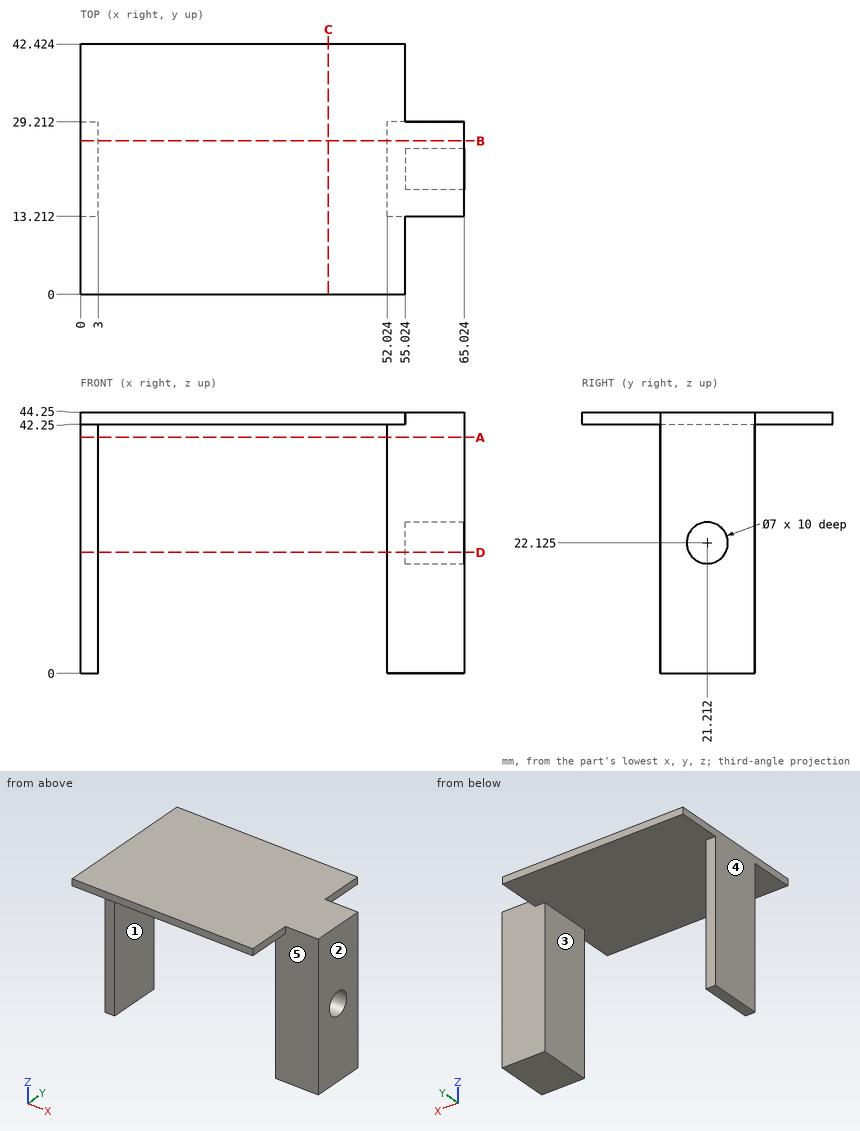
Check sheet for the drawn part. Datum: minimum x, y, z corner. Units: mm. A direction names the side the tool comes from. Give positions to 0.01 mm unless a question says otherwise; leave off trailing zeros. Write each loop counter-clockwise with the first axis right and the second up, starting at its lowest first coordinate (ties: lowest second). Pieces come first, ordered by that corner, then holes. Notation, with made-up numbers: (41.25, -9) -> (48.25, -9) arc R17 ccw to (48.25, 4) -> close; hole circle Ø9 at (63.5, -28). An arc over 180 degrees is marked (long way). Use one line per item in the form item = value. Start each with the question number.
1. Access from +Z, -Z, +X, -X, +Y, -Y to the whole of each face (thin tool, end or side, straight path). Record for the marked faces 1 and 2.
2. Section check A-A (z = 40). Record the cut outline in (x, y).
3. Thickness scan on line 1 along X through (y, z) = (22, 11.5); line 2 along Y through (x, z) = (60, 26); line 3 along Z through (x, y) = (44, 25). Record the ranges inside material, lowest first. Write a range as from..to.
4. Section check B-B (y = 26). Record the cut outline in (x, z).
5. Section check C-C (x = 42). Record the cut outline in (y, z).
6. Mould release check, pull along X, two halves, no side actions. Record for the marked faces 3, 4 and 5: pulls with the +X half, pulls with the -X half, needs draft (parallel to the pull), parting line crosses it, or undercut.
7. Section check D-D (z = 20.5). Record the cut outline in (x, y).
8. Go/stop test with flat-tipped pins: P1, Ø1.6, axis at y = 4, z = 43.5, coming from the +X side; P2, Ø6.5, axis at x = 57.5, z = 31.5, coming from the -Y side; P3, Ø1.5, axis at x = 2, z = 11.5, coming from the +Y side; P4, Ø12, axis at x = 40.5, z = 6, coming from the -Y side. Record where each tip stops, or that it passes through.
Conclusion:
q1.face_1 = -Z, +Y, -Y
q1.face_2 = +Z, -Z, +X, +Y, -Y
q2.outline = (0, 13.21) -> (3, 13.21) -> (3, 29.21) -> (0, 29.21) -> close; (52.02, 13.21) -> (65.02, 13.21) -> (65.02, 29.21) -> (52.02, 29.21) -> close
q3.line_1 = 0..3, 52.02..65.02
q3.line_2 = 13.21..29.21
q3.line_3 = 42.25..44.25
q4.outline = (0, 0) -> (3, 0) -> (3, 42.25) -> (52.02, 42.25) -> (52.02, 0) -> (65.02, 0) -> (65.02, 44.25) -> (0, 44.25) -> close
q5.outline = (0, 42.25) -> (42.42, 42.25) -> (42.42, 44.25) -> (0, 44.25) -> close
q6.face_3 = undercut
q6.face_4 = pulls with the -X half
q6.face_5 = needs draft
q7.outline = (0, 13.21) -> (3, 13.21) -> (3, 29.21) -> (0, 29.21) -> close; (52.02, 13.21) -> (65.02, 13.21) -> (65.02, 18.11) -> (55.02, 18.11) -> (55.02, 24.31) -> (65.02, 24.31) -> (65.02, 29.21) -> (52.02, 29.21) -> close
q8.P1 = 55.02
q8.P2 = 13.21
q8.P3 = 29.21
q8.P4 = through
